```python
from build123d import *

# Parameters (mm, degrees)
F0_W     = 30
F0_H     = 30
F1_DEPTH = 960
F2_R     = 7.5
F3_DEPTH = 30.001
F4_R     = 5


with BuildPart() as f1:
    # F0 (on Top) → F1 (new body)
    with BuildSketch(Plane.XY):
        Rectangle(F0_W, F0_H)
    extrude(amount=F1_DEPTH)

    # F2 (on face) → F3 (cut, through all)
    with BuildSketch(Plane.YZ.offset(15)):
        with Locations((0, 30)):
            Circle(F2_R)
        with Locations((0, 92)):
            Circle(F2_R)
        with Locations((0, 154)):
            Circle(F2_R)
        with Locations((0, 216)):
            Circle(F2_R)
        with Locations((0, 278)):
            Circle(F2_R)
        with Locations((0, 340)):
            Circle(F2_R)
        with Locations((0, 402)):
            Circle(F2_R)
        with Locations((0, 464)):
            Circle(F2_R)
        with Locations((0, 526)):
            Circle(F2_R)
        with Locations((0, 588)):
            Circle(F2_R)
        with Locations((0, 650)):
            Circle(F2_R)
        with Locations((0, 712)):
            Circle(F2_R)
        with Locations((0, 774)):
            Circle(F2_R)
        with Locations((0, 836)):
            Circle(F2_R)
        with Locations((0, 898)):
            Circle(F2_R)
        with Locations((0, 960)):
            Circle(F2_R)
        with Locations((0, 1022)):
            Circle(F2_R)
        with Locations((0, 1084)):
            Circle(F2_R)
        with Locations((0, 1146)):
            Circle(F2_R)
        with Locations((0, 1208)):
            Circle(F2_R)
        with Locations((0, 1270)):
            Circle(F2_R)
        with Locations((0, 1332)):
            Circle(F2_R)
        with Locations((0, 1394)):
            Circle(F2_R)
        with Locations((0, 1456)):
            Circle(F2_R)
        with Locations((0, 1518)):
            Circle(F2_R)
        with Locations((0, 1580)):
            Circle(F2_R)
        with Locations((0, 1642)):
            Circle(F2_R)
        with Locations((0, 1704)):
            Circle(F2_R)
    extrude(amount=-F3_DEPTH, mode=Mode.SUBTRACT)

    # F4
    f4_edges = [f1.edges().sort_by_distance(p)[0] for p in [
        (15, -15, 480),
        (-15, -15, 480),
        (15, 15, 480),
        (-15, 15, 480),
    ]]
    fillet(f4_edges, radius=F4_R)


solid = f1.part
```
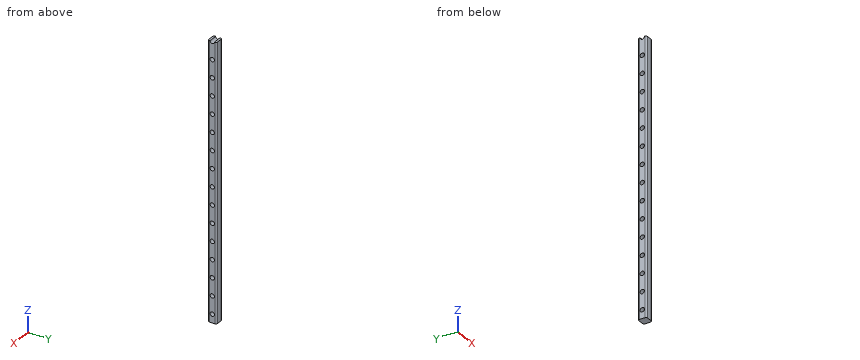
Could you check a few things on this model? Use its own coordinates, in mm. Coordinates: 2 decimals unless noted, no trailing zeros. Order: outer loops, then holes, each group sorted by start corner. A loop starts at its lowest first (then second) coordinate and runs counter-clockwise, first axis right, second up. Notation, with made-up numbers: M 39,6 L 66,6 A33 ccw 66,44 Z; hole C 47,-7 d1. An arc over 180 degrees is marked long. Use a Markdown table: item, result. Add a question column.
Q1. I'm going to push a flat-ended pin straight in: pin 1 (9 mm diameter, centred on y = 0, z = 526, fed in from +X). Where does the tip first touch, or does it pass through?
Q2. I want a section at B-B on z = 863. List the corners of the cut face in (x, y) for me.
Q3. I want a section at A-A on y = 0. Give the number of separate pieces and of enclosed holes in the cut face, then the cut area to 3 significant figures.
Q4. If I drill on L1, parallel to Y at x = -8.5, z = 650; L2, parallel to X at y = 11, z = 806.5; L3, parallel to Y at x = -9, z = 775.5, over which ranges is the centre line in solid material (lowest first)?
Checked values:
| question | item | result |
|---|---|---|
| 1 | pin 1 | through |
| 2 | outline | M -15,-10 A5 ccw -10,-15 L 10,-15 A5 ccw 15,-10 L 15,10 A5 ccw 10,15 L -10,15 A5 ccw -15,10 Z |
| 3 | separate pieces | 16 |
| 3 | enclosed holes | 0 |
| 3 | area | 21,800 mm² |
| 4 | L1 | -15 to -7.5, 7.5 to 15 |
| 4 | L2 | -14.9 to 14.9 |
| 4 | L3 | -15 to -7.35, 7.35 to 15 |
